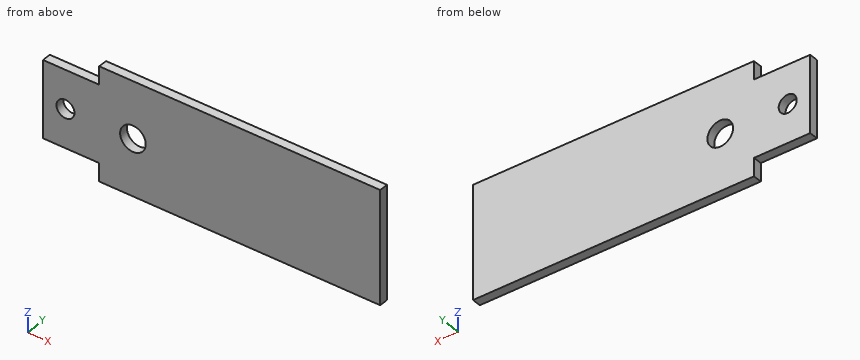
from build123d import *

# Parameters (mm, degrees)
SKETCH1_W           = 150
SKETCH1_H           = 50
BOSS_EXTRUDE1_DEPTH = 4
SKETCH2_R           = 4
SKETCH2_R_2         = 5.7
CUT_EXTRUDE1_DEPTH  = 4
SKETCH3_W           = 25
SKETCH3_H           = 8
CUT_EXTRUDE2_DEPTH  = 4


with BuildPart() as part:
    # Sketch1 → Boss-Extrude1 (new body)
    with BuildSketch(Plane(origin=(0, 0, 0), x_dir=(1, 0, 0), z_dir=(0, 1, 0))):
        Rectangle(SKETCH1_W, SKETCH1_H)
    extrude(amount=BOSS_EXTRUDE1_DEPTH)

    # Sketch2 → Cut-Extrude1 (cut)
    with BuildSketch(Plane.XZ):
        with Locations(Location((-65, 0, 0), (0, 0, 270))):
            Circle(SKETCH2_R)
        with Locations(Location((-35, 0, 0), (0, 0, 270))):
            Circle(SKETCH2_R_2)
    extrude(amount=-CUT_EXTRUDE1_DEPTH, mode=Mode.SUBTRACT)

    # Sketch3 → Cut-Extrude2 (cut)
    with BuildSketch(Plane(origin=(0, 4, 0), x_dir=(1, 0, 0), z_dir=(0, 1, 0))):
        with Locations((-62.5, 21)):
            Rectangle(SKETCH3_W, SKETCH3_H)
        with Locations((-62.5, -21)):
            Rectangle(SKETCH3_W, SKETCH3_H)
    extrude(amount=-CUT_EXTRUDE2_DEPTH, mode=Mode.SUBTRACT)


solid = part.part
For this review, take the finished solid that the model builds, in its own axes (mm). Give positions to 0.01 mm unless a question says otherwise; leave off trailing zeros. Loops run counter-clockwise (first coordinate to the right, second up) from the corner with the lowest first, then second, coordinate; pieces in that order, holes last. Notation, with made-up numbers: M 17.25,43.5 L 24.25,43.5 A16 ccw 24.25,57.5 Z; hole C 64.25,86 d9. An arc over 180 degrees is marked long. Put each result on its own line as item: value. Start each with the question number.
(1) For pin 1 (2 mm diameter, centred on x = -66.5, y = 1, fed in from +Z), flat-tipped, find the tip position at first contact; note if it passes through.
(2) Add section A-A, the plane z = 0. Write out the cut boundary in (x, y).
(3) Add section B-B, the plane x = -65. Write out the cut boundary in (y, z).
(4) Add section C-C, the plane y = 2.95. Write out the cut boundary in (x, z), then the cut area to 3 significant figures.
(5) Add section D-D, the plane x = -35. Write out the cut boundary in (y, z).
(6) Wall thickness on L1, parallel to X at y = 1.6, z = 0; L2, parallel to X at y = 0.9, z = 20; L3, parallel to Z at x = -38.5, y = 1.8: over which ranges is each line inside the solid? List them lowest first.
Result:
1. pin 1: stops at z = 17
2. outline: M -75,0 L -69,0 L -69,4 L -75,4 Z; M -61,0 L -40.7,0 L -40.7,4 L -61,4 Z; M -29.3,0 L 75,0 L 75,4 L -29.3,4 Z
3. outline: M 0,-17 L 4,-17 L 4,-4 L 0,-4 Z; M 0,4 L 4,4 L 4,17 L 0,17 Z
4. outline: M -75,-17 L -50,-17 L -50,-25 L 75,-25 L 75,25 L -50,25 L -50,17 L -75,17 Z; hole C -65,0 d8; hole C -35,0 d11.4
4. area: 6,950 mm^2
5. outline: M 0,-25 L 4,-25 L 4,-5.7 L 0,-5.7 Z; M 0,5.7 L 4,5.7 L 4,25 L 0,25 Z
6. L1: x = -75 to -69, -61 to -40.7, -29.3 to 75
6. L2: x = -50 to 75
6. L3: z = -25 to -4.5, 4.5 to 25
